CAD build for the part. Positions are in the model's coordinates, mm. A direction names the side the tool comes from. Round coordinates to 2 decimals unless told otherwise and drop trailing zeros. Loops run counter-clockwise (first coordinate to the right, second up) from the corner with the lowest first, then second, coordinate; pieces in that order, holes last. Notation, with made-up numbers: M 66,70 L 88,70 A22 ccw 88,106 Z; hole C 4,60 d1. An arc over 180 degrees is marked long. Use a Markdown table: item, result. Add a question column.
(1) Two-plate mould, pull along Z, no slides. Class faces 3 (the face through (-37, 25, 5)), 4 (the face through (-31.036, 12.325, 42.375)), 5 (the face through (0, 13, -37.829)), 6 (the face through (0, 12, -39.829)): released by +Z, released by -Z, zero draft, split by the parting line, or undercut.
(2) Flat gauge pins, fed straight in: P1, Ø3, axis at x = 27.5, y = 13.5, coming from the -Z side; P2, Ø1, axis at y = 6.5, z = 6.5, coming from the +X side; P3, Ø21.5, axis at x = -7.5, z = 19.5, coming from the +Y side. Where does each tip first touch, or does it go through?
(3) Wall check: L1, parallel to X at y = 7.25, z = 33; L2, parallel to X at y = 24.25, z = -23; L3, parallel to Z at x = 22, y = 5.5. Give the ranges that are in metal, low to high.
(4) Which spindle directions (+Z, -Z, +X, -X, +Y, -Y) get a long thin tool onto all of the face, cutting with end or side? Do faces 1 (the face through (30.04, 13.34, -30.71)), 2 (the face through (-31.52, 12.32, -32.06)). Say none if no direction does.
(5) Band-saw the part on C-C, the plane z = -17.5. Write the cut outline in (x, y), and give its area (3 significant figures).
(6) Band-saw the part on B-B, the plane x = 11.5. Write the cut outline in (y, z), and give its area (3 significant figures).
(7) Band-saw the part on A-A, the plane y = 8. Write the cut outline in (x, z).
from build123d import *

# Parameters (mm, degrees)
AUFSATZ_LINEAR_AUSTRAGEN1_DEPTH = 25
WANDUNG2_T                      = -2


with BuildPart() as part:
    # Skizze1 → Aufsatz-Linear austragen1 (new body)
    with BuildSketch(Plane(origin=(0, 0, 0), x_dir=(1, 0, 0), z_dir=(0, 1, 0))):
        Polygon((0, -50.171355376), (-25, -50.171355376), (-37.244282987, -34.357515421), (-37.855752194, 24.507755761), (-25, 39.828644624), (0, 39.828644624), align=None)
    aufsatz_linear_austragen1 = extrude(amount=AUFSATZ_LINEAR_AUSTRAGEN1_DEPTH)

    # Spiegeln1: Aufsatz-Linear austragen1 across plane
    add(aufsatz_linear_austragen1.mirror(Plane(origin=(0, 0, 0), x_dir=(0, 0, 1), z_dir=(1, 0, 0))))

    # Wandung2
    wandung2_openings = [part.faces().sort_by_distance(p)[0] for p in [
        (0, 25, 5.030518753),
    ]]
    offset(amount=WANDUNG2_T, openings=wandung2_openings, kind=Kind.INTERSECTION)


solid = part.part
Return value:
| question | item | result |
|---|---|---|
| 1 | face 3 | zero draft |
| 1 | face 4 | released by +Z |
| 1 | face 5 | undercut |
| 1 | face 6 | released by -Z |
| 2 | P1 | z = -38.64 |
| 2 | P2 | x = 37.54 |
| 2 | P3 | y = 2 |
| 3 | L1 | -37.26 to -35.26, 35.26 to 37.26 |
| 3 | L2 | -37.84 to -35.84, 35.84 to 37.84 |
| 3 | L3 | -39.83 to -37.83, 48.17 to 50.17 |
| 4 | face 1 | +Y |
| 4 | face 2 | -Z, -X, +Y, -Y |
| 5 | outline | M -37.78,0 L 37.78,0 L 37.78,25 L 35.78,25 L 35.78,2 L -35.78,2 L -35.78,25 L -37.78,25 Z |
| 5 | area | 243 mm^2 |
| 6 | outline | M 0,-39.83 L 25,-39.83 L 25,-37.83 L 2,-37.83 L 2,48.17 L 25,48.17 L 25,50.17 L 0,50.17 Z |
| 6 | area | 272 mm^2 |
| 7 | outline | M -37.86,-24.51 L -25,-39.83 L 25,-39.83 L 37.86,-24.51 L 37.24,34.36 L 25,50.17 L -25,50.17 L -37.24,34.36 Z; hole M -35.85,-23.79 L -24.07,-37.83 L 24.07,-37.83 L 35.85,-23.79 L 35.25,33.66 L 24.02,48.17 L -24.02,48.17 L -35.25,33.66 Z |
